from build123d import *

# Parameters (mm, degrees)
F0_W     = 457.2
F0_H     = 584.2
F1_DEPTH = 19.05
F2_W     = 19.05
F2_H     = 584.2
F3_DEPTH = 6.35
F4_W     = 419.1
F4_H     = 12.7
F5_DEPTH = 6.35


with BuildPart() as f1:
    # F0 (on Top) → F1 (new body)
    with BuildSketch(Plane.XY):
        with Locations((0, -12.7)):
            Rectangle(F0_W, F0_H)
    extrude(amount=F1_DEPTH)

    # F2 (on face) → F3 (cut)
    with BuildSketch(Plane.XY.offset(19.05)):
        with Locations((219.075, -12.7)):
            Rectangle(F2_W, F2_H)
        with Locations((-219.075, -12.7)):
            Rectangle(F2_W, F2_H)
    extrude(amount=-F3_DEPTH, mode=Mode.SUBTRACT)

    # F4 (on face) → F5 (cut)
    with BuildSketch(Plane.XY.offset(19.05)):
        with Locations((0, 273.05)):
            Rectangle(F4_W, F4_H)
    extrude(amount=-F5_DEPTH, mode=Mode.SUBTRACT)


solid = f1.part
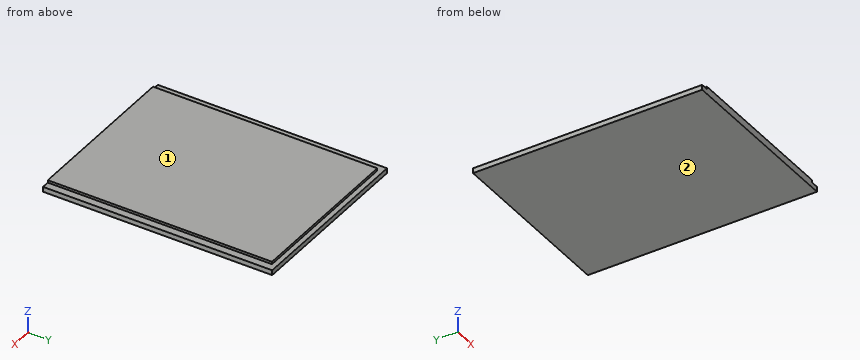
Source: CAD feature listing. Evaluate the final solid. Frame: model axes, mm. Face numbers are marked on the shaded views. Give positions to 0.01 mm unless a question says otherwise; leave off trailing zeros. Write each loop counter-clockwise with the first axis right and the second up, starting at its lowest first coordinate (ties: lowest second). Pieces come first, ordered by that corner, then holes. Notation, with made-up numbers: (23, 22) -> (29, 22) arc R16 ccw to (29, 36) -> close; hole circle Ø2 at (-32.5, 58). An arc over 180 degrees is marked (long way). Write item = value, one per line.
Q1. First-contact query: pin 1 (1.9 mm diameter, centred on x = -57.5, z = 14.5, fed in from +Y). Flat tip, straight axial feed; report the tip coordinate or a pass-through.
Here are the results:
pin_1 = 266.7
Q2. Cut plane A-A on y = -200. Return loops of the section in (x, z).
Here are the results:
outline = (-228.6, 0) -> (228.6, 0) -> (228.6, 12.7) -> (209.55, 12.7) -> (209.55, 19.05) -> (-209.55, 19.05) -> (-209.55, 12.7) -> (-228.6, 12.7) -> close
Q3. Mould query, pull axis Z, two halves, no side actions, for the marked faces 1 and 2. Classes: +Z half, -Z half, draft (parallel to the pull), parting line (faces both ways), or undercut.
Here are the results:
face_1 = +Z half
face_2 = -Z half
Q4. Line query: line 1 (X direction, y = -196, z = 16.75); line 2 (Y direction, x = -199.5, z = 13). Output: solid intervals per line, ascending. Write a range as from..to.
Here are the results:
line_1 = -209.55..209.55
line_2 = -304.8..266.7
